```python
from build123d import *

# Parameters (mm, degrees)
PAD_DEPTH       = 9
POCKET_DEPTH    = 10
POCKET001_DEPTH = 5
SKETCH003_R     = 1.6
POCKET002_DEPTH = 5
POCKET003_DEPTH = 2


with BuildPart() as part:
    # Sketch → Pad (new body)
    with BuildSketch(Plane.XY):
        Polygon((-21, 41.246133918), (21, 52.5), (21, -52.5), (-21, -52.5), align=None)
    extrude(amount=PAD_DEPTH)

    # Sketch001 → Pocket (cut)
    with BuildSketch(Plane.XY.offset(9)):
        Polygon((-19.5, 40.095143436), (-19.5, -10.619723875), (19.5, 11.8969366233), (19.5, 50.5451619407), align=None)
        Polygon((-19.5, -12.3517746826), (-19.5, -51), (19.5, -51), (19.5, 10.1648858158), align=None)
    extrude(amount=-POCKET_DEPTH, mode=Mode.SUBTRACT)

    # Sketch002 → Pocket001 (cut)
    with BuildSketch(Plane(origin=(-11.7182667397, 43.7331668494, 0), x_dir=(-0.9659258263, -0.2588190451, 0), z_dir=(-0.2588190451, 0.9659258263, 0))):
        with BuildLine():
            ThreePointArc((-2.8908426427, 6.15), (-4.5408426427, 4.5), (-2.8908426427, 2.85))
            Line((-2.8908426427, 2.85), (3.6091573573, 2.85))
            ThreePointArc((3.6091573573, 2.85), (5.2591573573, 4.5), (3.6091573573, 6.15))
            Line((-2.8908426427, 6.15), (3.6091573573, 6.15))
        make_face()
        with BuildLine():
            ThreePointArc((-29.8908426427, 6.15), (-31.5408426427, 4.5), (-29.8908426427, 2.85))
            Line((-29.8908426427, 2.85), (-23.3908426427, 2.85))
            ThreePointArc((-23.3908426427, 2.85), (-21.7408426427, 4.5), (-23.3908426427, 6.15))
            Line((-29.8908426427, 6.15), (-23.3908426427, 6.15))
        make_face()
    extrude(amount=-POCKET001_DEPTH, mode=Mode.SUBTRACT)

    # Sketch003 → Pocket002 (cut)
    with BuildSketch(Plane.XY.offset(9)):
        with Locations((37, -21.7740142833)):
            Circle(SKETCH003_R)
    extrude(amount=-POCKET002_DEPTH, mode=Mode.SUBTRACT)

    # Sketch004 → Pocket003 (cut)
    with BuildSketch(Plane.YZ.offset(21)):
        with BuildLine():
            ThreePointArc((-47.5, 6.15), (-49.15, 4.5), (-47.5, 2.85))
            Line((-47.5, 2.85), (-42.5, 2.85))
            ThreePointArc((-42.5, 2.85), (-40.85, 4.5), (-42.5, 6.15))
            Line((-47.5, 6.15), (-42.5, 6.15))
        make_face()
    extrude(amount=-POCKET003_DEPTH, mode=Mode.SUBTRACT)


solid = part.part
```
Input: part model. Units: mm. Frame: model coordinates. A direction names the side the tool comes from. Give positions to 0.01 mm unless a question says otherwise; leave off trailing zeros. Order: outer loops, then holes, each group sorted by start corner. A loop starts at its lowest first (then second) coordinate and runs counter-clockwise, first axis right, second up. Notation, with made-up numbers: (74.5, -30) - (107.5, -30) arc R8 cw to (107.5, -26) - close; hole circle Ø1 at (19, -35.5). An arc over 180 degrees is marked (long way). One line per item, written item: value.
1. Reachability of faces 5 (the face through (-21, -6, 4)), 6 (the face through (19.5, -21, 5)), 7 (the face through (18.94, 51.18, 4.54)), 8 (the face through (-12, 43, 6.15)), 9 (the face through (-0.294, 46.794, 4.437)) from +Z, -Z, +X, -X, +Y, -Y: full face, straight path, thin tool, end or side. Return the list, or none.
Determined:
face 5: +Z, -Z, -X, +Y, -Y
face 6: +Z, -Z
face 7: -X
face 8: +Y
face 9: +Z, -Z, -X, +Y
2. Draft query along Z for faces 1 (the face through (1.7, 0.2, 9)), 2 (the face through (0, -51, 5)), 3 (the face through (-7.14, 44.19, 4.54)), 4 (the face through (19.793, 47.994, 4.52)). Return one class per face: released by +Z, released by -Z, zero draft, split by the parting line, or undercut.
Determined:
face 1: released by +Z
face 2: zero draft
face 3: undercut
face 4: undercut
3. Cut plane A-A, the plane z = 1.5. Output: boundary loops of the cut face in (x, y).
Determined:
outline: (-21, -52.5) - (21, -52.5) - (21, 52.5) - (-21, 41.25) - close; hole (-19.5, -51) - (19.5, -51) - (19.5, 10.16) - (-19.5, -12.35) - close; hole (-19.5, -10.62) - (19.5, 11.9) - (19.5, 50.55) - (-19.5, 40.1) - close
4. Pin query (flat end, axial travel): pin 1 Ø3 at (x, z) = (-15.5, 2.5) entering from +Y; pin 2 Ø4 at (x, z) = (-4.5, 2.5) entering from +Y. Return the tip coordinate at first contact, or that it passes through.
Determined:
pin 1: y = 43.12
pin 2: y = 46.2
5. Cut plane C-C, the plane x = 2.5. Output: boundary loops of the cut face in (y, z).
Determined:
outline: (-52.5, 0) - (-51, 0) - (-51, 9) - (-52.5, 9) - close; (0.35, 0) - (2.08, 0) - (2.08, 9) - (0.35, 9) - close; (45.99, 0) - (47.54, 0) - (47.54, 9) - (45.99, 9) - close
6. Line query: probe 1 along X at (y, z) = (-20, 6.5); probe 2 along X at (y, z) = (-7, 1.5); probe 3 along Y at (x, z) = (-2, 3). Output: solid intervals per line, ascending.
Determined:
probe 1: -21 to -19.5, 19.5 to 21
probe 2: -21 to -19.5, -13.23 to -10.23, 19.5 to 21
probe 3: -52.5 to -51, -2.25 to -0.52, 44.78 to 46.34
7. Cut plane B-B, the plane y = 35.5. Output: boundary loops of the cut face in (x, z), and give its area (3 significant figures).
Determined:
outline: (-21, 0) - (-19.5, 0) - (-19.5, 9) - (-21, 9) - close; (19.5, 0) - (21, 0) - (21, 9) - (19.5, 9) - close
area: 27.0 mm2
